Read the model definition and answer for the solid it produces. Units are mm, in the model's axes. Face numbers are marked on the shaded views. A direction names the side the tool comes from. Coordinates: 2 decimals unless noted, no trailing zeros. Write each loop counter-clockwise with the first axis right and the second up, starting at its lowest first coordinate (ties: lowest second). Pieces come first, ordered by that corner, then holes.
1) The part is cut by section B-B (z = -49). Determine the outline of the cut face in (x, y) (3 decimals), then the cut area to 3 significant figures.
2) Which of the six approach directions +Z, -Z, +X, -X, +Y, -Y give full straight-line access (tool end or side, diameter ignored) to the marked faces 1 and 2?
3) The part is cut by section A-A (y = 0). Determine the outline of the cut face in (x, z) (1 decimal).
4) Find the intervals of material crossed by line 1 (Z direction, x = -2, y = -4.75); line 2 (Z direction, x = -1, y = 0.5); line 3 (Y direction, x = -0.25, z = -34), in increasing order.
5) Each of these flat-tipped pins is pushed along its axis until it touches: pin 1 Ø1.1 at (y, z) = (-0.5, -1) entering from +X; pin 2 Ø6 at (x, z) = (0.5, -64.5) entering from +Y (3 decimals); pin 3 Ø8 at (y, z) = (-1, -41) entering from +X (3 decimals). Where does it stop, or does it pass through?
from build123d import *

# Parameters (mm, degrees)
SKETCH1_W           = 76.2
SKETCH1_H           = 3.175
CHAMFER1_SIZE       = 0.9525
CUT_EXTRUDE2_DEPTH  = 2.86258
BOSS_EXTRUDE2_START = -45.722795596
SKETCH9_R           = 3.175
BOSS_EXTRUDE2_DEPTH = 45.722795596


with BuildPart() as part:
    # Sketch1 → Revolve1 (revolve)
    with BuildSketch(Plane(origin=(0, 0, 0), x_dir=(0, 0, -1), z_dir=(1, 0, 0))):
        with Locations((38.1, 1.5875)):
            Rectangle(SKETCH1_W, SKETCH1_H)
    revolve(axis=Axis((0, 0, -76.2), (0, 0, 1)))

    # Chamfer1
    chamfer1_edges = [part.edges().sort_by_distance(p)[0] for p in [
        (0, -3.175, -76.2),
    ]]
    chamfer(chamfer1_edges, length=CHAMFER1_SIZE)

    # Sketch7 → Revolve2 (revolve)
    with BuildSketch(Plane(origin=(0, 0, 0), x_dir=(0, 0, -1), z_dir=(1, 0, 0)), mode=Mode.PRIVATE) as revolve2_sk:
        with BuildLine():
            Line((0, 6.7437), (0.40894, 6.7437))
            Line((0.40894, 6.7437), (4.0894, 3.544324933))
            ThreePointArc((4.0894, 3.544324933), (4.549909788, 3.270350399), (5.077204404, 3.175))
            Line((5.077204404, 3.175), (5.077204404, 0))
            Line((5.077204404, 0), (0, 0))
            Line((0, 0), (0, 6.7437))
        make_face()
    revolve(revolve2_sk.sketch.rotate(Axis((0, 0, 0), (0, 0, -1)), 180), axis=Axis((0, 0, 0), (0, 0, -1)))

    # Boss-Extrude1 cone 1 section (through the dimple's axis) → Boss-Extrude1 (revolve)
    with BuildSketch(Plane(origin=(0, 0, -5.077204404), x_dir=(0, -1, 0), z_dir=(1, 0, 0))):
        Polygon((0, 0), (3.175, 0), (0, 3.175), align=None)
    revolve(axis=Axis((0, 0, -5.077204404), (0, 0, -1)))

    # Sketch5 → Cut-Extrude2 (cut)
    with BuildSketch(Plane.XY):
        Polygon((1.984375, -1.14567944), (1.984375, 1.14567944), (0, 2.291358881), (-1.984375, 1.14567944), (-1.984375, -1.14567944), (0, -2.291358881), align=None)
    extrude(amount=-CUT_EXTRUDE2_DEPTH, mode=Mode.SUBTRACT)

    # Cut-Extrude3 cone 1 section (through the dimple's axis) → Cut-Extrude3 (revolve, cut)
    with BuildSketch(Plane(origin=(0, 0, 0), x_dir=(0, -1, 0), z_dir=(1, 0, 0))):
        Polygon((0, 0), (2.291358881, 0), (0, 2.291358881), align=None)
    revolve(axis=Axis((0, 0, 0), (0, 0, -1)), mode=Mode.SUBTRACT)

    # Sketch9 → Boss-Extrude2 (add)
    with BuildSketch(Plane.XY.offset(-5.077204404).offset(BOSS_EXTRUDE2_START)):
        with Locations(Location((0, 0, 0), (0, 0, 90))):
            Circle(SKETCH9_R)
    extrude(amount=BOSS_EXTRUDE2_DEPTH)


solid = part.part
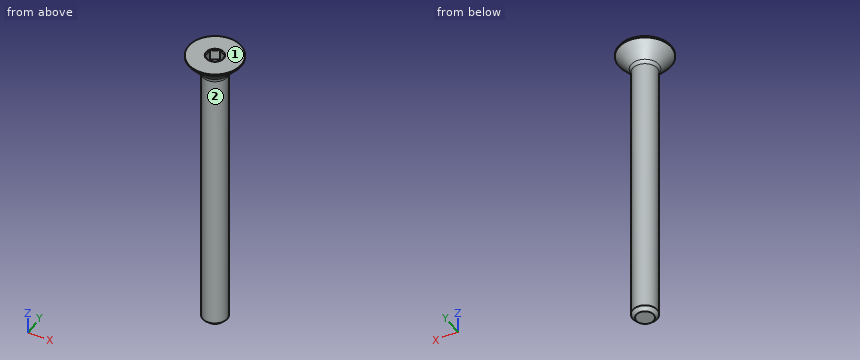
Reported:
1. outline: circle Ø6.35 at (0, 0)
1. area: 31.7 mm2
2. face 1: +Z, +X, -X, +Y, -Y
2. face 2: -Z
3. outline: (-6.7, -0.4) - (-3.5, -4.1) arc R1.5 cw to (-3.2, -5.1) - (-3.2, -75.2) - (-2.2, -76.2) - (2.2, -76.2) - (3.2, -75.2) - (3.2, -5.1) arc R1.5 cw to (3.5, -4.1) - (6.7, -0.4) - (6.7, 0) - (2.3, 0) - (2, -0.3) - (2, -2.9) - (-2, -2.9) - (-2, -0.3) - (-2.3, 0) - (-6.7, 0) - close
4. line 1: z = -2.24 to 0
4. line 2: z = -76.2 to -2.86
4. line 3: y = -3.17 to 3.17
5. pin 1: stops at x = 6.69
5. pin 2: stops at y = 3.175
5. pin 3: stops at x = 3.175
